Job drawing, mm, ordinate dimensions from the low corner. One solid piece. Round coordinates to 2 decimals unless told otherwise and drop trailing zeros. Loops run counter-clockwise (first coordinate to the right, second up) from the corner with the lowest first, then second, coordinate; pieces in that order, holes last.
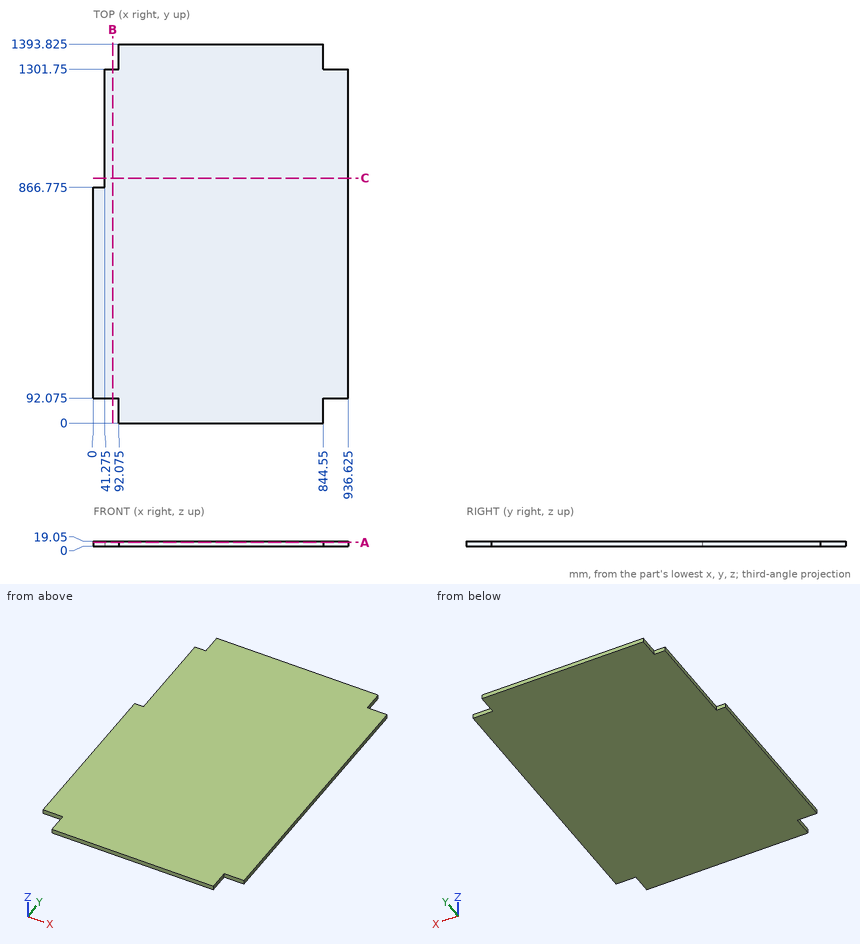
Item 1: Cut at A-A, the plane z = 15. Give the cut face in (x, y) (3 decimals).
Answers follow:
outline: (0, 92.075) - (92.075, 92.075) - (92.075, 0) - (844.55, 0) - (844.55, 92.075) - (936.625, 92.075) - (936.625, 1301.75) - (844.55, 1301.75) - (844.55, 1393.825) - (92.075, 1393.825) - (92.075, 1301.75) - (41.275, 1301.75) - (41.275, 866.775) - (0, 866.775) - close
Item 2: Flat gauge pins, fed straight in: P1, Ø9.5, axis at x = 14.5, z = 13.5, coming from the +Y side (3 decimals); P2, Ø9.5, axis at x = 910.5, z = 12.5, coming from the +Y side; P3, Ø5.5, axis at y = 1356.5, z = 12, coming from the -X side (3 decimals). Where does each tip first touch, or does it go through?
Answers follow:
P1: stops at y = 866.775
P2: stops at y = 1301.75
P3: stops at x = 92.075
Item 3: Probe line 1 (X direction, y = 1170, z = 15.5) (3 decimals); line 2 (X direction, y = 1335.5, z = 13) (3 decimals); line 3 (Y direction, x = 864.5, z = 14) (3 decimals). List the from-to ranges inside material, lowest first.
Answers follow:
line 1: x = 41.275 to 936.625
line 2: x = 92.075 to 844.55
line 3: y = 92.075 to 1301.75
Item 4: Cut at B-B, the plane x = 70.5. Give the cut face in (y, z) (3 decimals), plus the area to 3 significant figures.
Answers follow:
outline: (92.075, 0) - (1301.75, 0) - (1301.75, 19.05) - (92.075, 19.05) - close
area: 23,000 mm2
Item 5: Cut at C-C, the plane y = 900.5. Give the cut face in (x, z) (3 decimals), plus the area to 3 significant figures.
Answers follow:
outline: (41.275, 0) - (936.625, 0) - (936.625, 19.05) - (41.275, 19.05) - close
area: 17,100 mm2
